Geometry: see drawing. Coordinates: mm, zero at the bounding-box minimum. A direction names the side the tool comes from. Round coordinates to 2 decimals unless told otherwise and drop trailing zeros. Order: outer loops, then holes, each group sorted by start corner. A loop starts at its lowest first (then second) coordinate and runs counter-clockwise, first axis right, second up. Notation, with made-up numbers: (20.25, 84) -> (75.25, 84) arc R8 cw to (75.25, 95) -> close; hole circle Ø1 at (-6, 57). An arc over 180 degrees is marked (long way). One line per item, written item: value. Start each with the question number.
1) Mould query, pull axis Y, two halves, no side actions, for the marked faces 1, 2 and 3. Classes: pulls with the +Y half, pulls with the -Y half, needs draft (parallel to the pull), parting line crosses it, or undercut.
2) Section D-D (x = 7.54). Return the cut outline in (y, z), and give its area (3 significant figures).
3) Reachability of the marked faces 4, 5, 6, 7 and 8 from +Z, -Z, +X, -X, +Y, -Y: full face, straight path, thin tool, end or side. Return the list, or none.
4) Section C-C (y = 6.25). Return the cut outline in (x, z), and give its area (3 significant figures).
5) Section B-B (x = 5). Return the cut outline in (y, z), and give its area (3 significant figures).
6) Ray query, L1, parallel to Y at x = 5.5, z = 15; L2, parallel to Z at x = 0.5, y = 7.5; L3, parallel to Z at x = 8, y = 6.5. Return the intervals inside material, ascending.
7) Section A-A (z = 18.5). Return the cut outline in (x, y), and give its area (3 significant figures).
8) Pin query (flat end, axial travel): P1, Ø1.2, axis at x = 7.5, y = 6.5, coming from the +Z side; P2, Ø1.5, axis at y = 3.5, z = 9, coming from the +X side. Return the tip coordinate at first contact, or that it passes through.
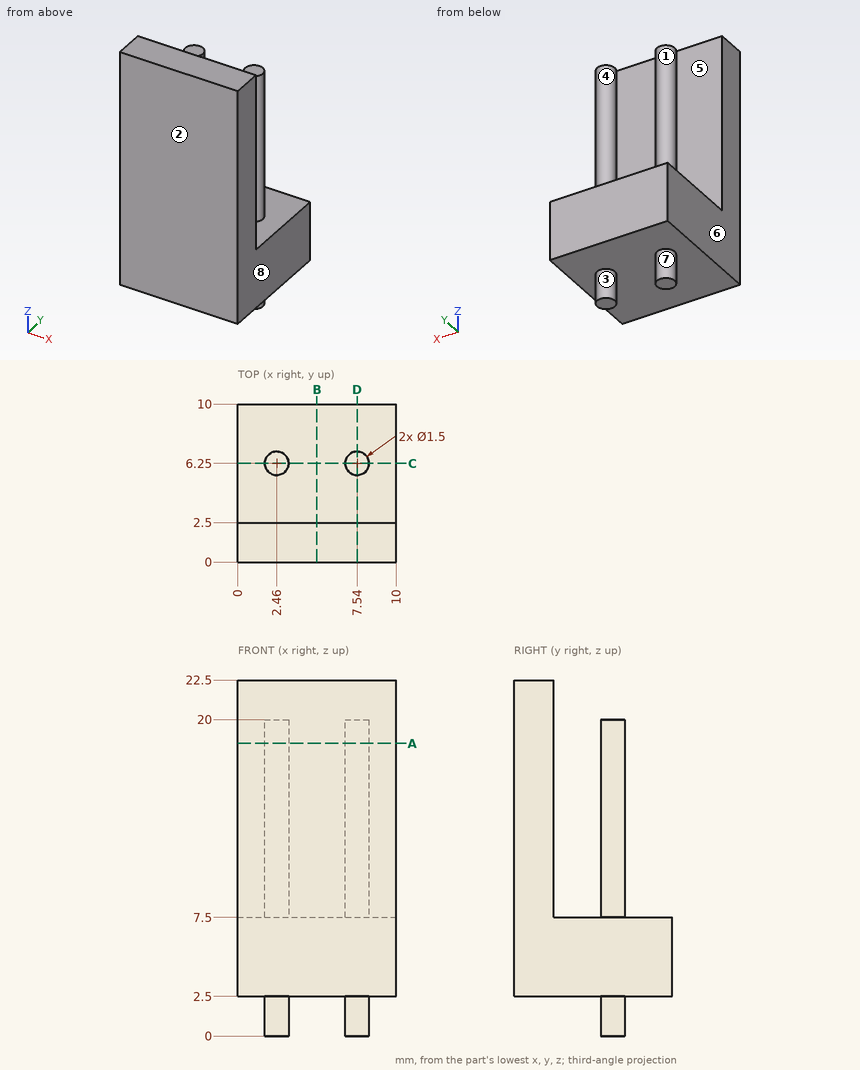
Findings:
1. face 1: undercut
1. face 2: pulls with the -Y half
1. face 3: parting line crosses it
2. outline: (0, 2.5) -> (5.5, 2.5) -> (5.5, 0) -> (7, 0) -> (7, 2.5) -> (10, 2.5) -> (10, 7.5) -> (7, 7.5) -> (7, 20) -> (5.5, 20) -> (5.5, 7.5) -> (2.5, 7.5) -> (2.5, 22.5) -> (0, 22.5) -> close
2. area: 110 mm2
3. face 4: +Z
3. face 5: +Z, +X, -X
3. face 6: +Z, -Z, -X, +Y, -Y
3. face 7: -Z
3. face 8: +Z, -Z, +X, +Y, -Y
4. outline: (0, 2.5) -> (1.71, 2.5) -> (1.71, 0) -> (3.21, 0) -> (3.21, 2.5) -> (6.79, 2.5) -> (6.79, 0) -> (8.29, 0) -> (8.29, 2.5) -> (10, 2.5) -> (10, 7.5) -> (8.29, 7.5) -> (8.29, 20) -> (6.79, 20) -> (6.79, 7.5) -> (3.21, 7.5) -> (3.21, 20) -> (1.71, 20) -> (1.71, 7.5) -> (0, 7.5) -> close
4. area: 95.0 mm2
5. outline: (0, 2.5) -> (10, 2.5) -> (10, 7.5) -> (2.5, 7.5) -> (2.5, 22.5) -> (0, 22.5) -> close
5. area: 87.5 mm2
6. L1: 0 to 2.5
6. L2: 2.5 to 7.5
6. L3: 0 to 20
7. outline: (0, 0) -> (10, 0) -> (10, 2.5) -> (0, 2.5) -> close; circle Ø1.5 at (2.46, 6.25); circle Ø1.5 at (7.54, 6.25)
7. area: 28.5 mm2
8. P1: z = 20
8. P2: through
